Autodesk Inventor part; units mm, degrees
ref_plane "YZ Plane" through (0, 0, 0) normal (1, 0, 0) x (0, 1, 0)
ref_plane "XZ Plane" through (0, 0, 0) normal (0, 1, 0) x (-1, 0, 0)
ref_plane "XY Plane" through (0, 0, 0) normal (0, 0, 1) x (1, 0, 0)
sketch "Sketch1" plane through (0, 0, 0) normal (0, 0, 1) x (1, 0, 0)
  circle A0 centre (0, 0) radius 101.6
  circle A1 centre (0, 0) radius 14.2875
  dimension "d0" = 203.2
  dimension "d1" = 28.575
extrude "Extrusion1" add sketch "Sketch1" along normal blind 4.7625
sketch "Sketch4" plane through (0, 0, 4.7625) normal (0, 0, 1) x (1, 0, 0)
  circle A0 centre (0, 0) radius 101.6
  circle A1 centre (0, 92.075) radius 2.8063
  line L0 (0, 0) -> (0, 101.6) construction
  circle A2 centre (0, 0) radius 92.075 construction
  dimension "d58" = 9.525
extrude "Extrusion5" cut sketch "Sketch4" against normal through all contours A1
pattern_circular "Circular Pattern3" count 24 over 360 about axis through (0, 0, -10) along (0, 0, 1) of "Extrusion5"
sketch "Sketch6" plane through (0, 0, 4.7625) normal (0, 0, 1) x (1, 0, 0)
  circle A0 centre (0, 0) radius 101.6
  circle A1 centre (0, 23.8125) radius 2.3813
  circle A2 centre (0, 0) radius 23.8125 construction
  line L0 (0, 23.8125) -> (0, 0) construction
  dimension "d68" = 47.625
  dimension "d69" = 4.7625
extrude "Extrusion6" cut sketch "Sketch6" against normal through all contours A1
pattern_circular "Circular Pattern4" count 6 over 360 about axis through (0, 0, -10) along (0, 0, 1) of "Extrusion6"
sketch "Sketch7" plane through (0, 0, 4.7625) normal (0, 0, 1) x (1, 0, 0)
  circle A0 centre (-20.6222, -11.9062) radius 2.3813
  circle A1 centre (-20.6222, 11.9062) radius 2.3813
  circle A2 centre (0, 23.8125) radius 2.3813
  circle A3 centre (0, 0) radius 101.6
  line L0 (0, 0) -> (0, 23.8125) construction
  line L1 (0, 23.8125) -> (0, 0) construction
  line L2 (-20.6222, 11.9062) -> (0, 0) construction
  line L3 (-20.6222, -11.9062) -> (0, 0) construction
  line L4 (-25.4, 5.4993) -> (-68.7895, 30.5502)
  line L5 (-68.7895, -30.5502) -> (-25.4, -5.4993)
  arc A4 (-77.9615, 27.1385) -> (-77.9615, -27.1385) centre (0, 0) ccw
  arc A5 (-68.7895, 30.5502) -> (-77.9615, 27.1385) centre (-71.9645, 25.0509) ccw
  arc A6 (-77.9615, -27.1385) -> (-68.7895, -30.5502) centre (-71.9645, -25.0509) ccw
  arc A7 (-25.4, -5.4993) -> (-25.4, 5.4993) centre (-28.575, 0) ccw
  point P0 (-75.1279, -34.2097)
  point P1 (-75.1279, 34.2097)
  dimension "d75" = 19.05
  dimension "d76" = 6.35
  dimension "d78" = 7.9375
extrude "Extrusion7" cut sketch "Sketch7" against normal through all contours A7 L5 A6 A4 A5 L4
pattern_circular "Circular Pattern5" count 6 over 360 about axis through (0, 0, -10) along (0, 0, 1) of "Extrusion7"
properties part number "FlyWheelBase" material "Aluminum-6061"
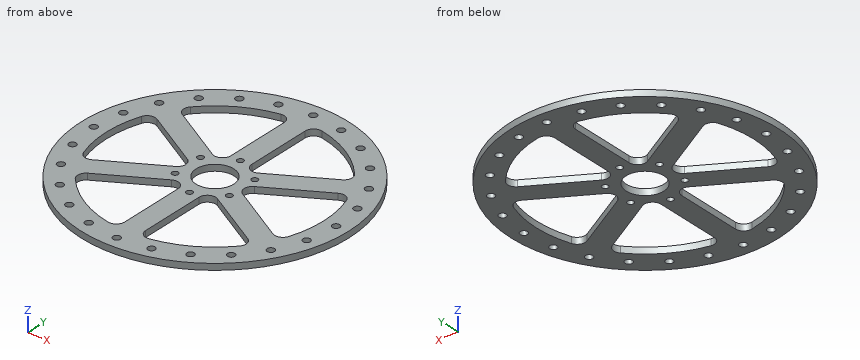
Geometry check sheet. Reference: the model listing, model coordinates, mm. Give positions to 0.01 mm unless a question says otherwise; leave off trailing zeros. Order: outer loops, then holes, each group sorted by start corner. A loop starts at its lowest first (then second) coordinate and runs counter-clockwise, first axis right, second up. Notation, with made-up numbers: M 8,47 L 60,47 A21 cw 60,55 Z; hole C -34.75,20 d9. An arc over 180 degrees is marked long. Use a Markdown table: item, result.
Item 1: Section check D-D (x = -36.5). Record the cut outline in (y, z).
Answers follow:
| item | result |
|---|---|
| outline | M -94.82,0 L -74.04,0 L -74.04,4.76 L -94.82,4.76 Z; M -30.24,0 L -11.91,0 L -11.91,4.76 L -30.24,4.76 Z; M 11.91,0 L 30.24,0 L 30.24,4.76 L 11.91,4.76 Z; M 74.04,0 L 94.82,0 L 94.82,4.76 L 74.04,4.76 Z |
Item 2: Material ranges on line 1 along Y through (x, z) = (-59.5, 2.3); line 2 along X through (y, z) = (-54, 2); line 3 along Y through (x, z) = (0, 2.25), recorded low to high.
Answers follow:
| item | result |
|---|---|
| line 1 | y = -82.35 to -57.22, -43.52 to -25.19, 25.19 to 43.52, 57.22 to 82.35 |
| line 2 | x = -86.06 to -62.44, -7.94 to 7.94, 62.44 to 86.06 |
| line 3 | y = -101.6 to -94.88, -89.27 to -26.19, -21.43 to -14.29, 14.29 to 21.43, 26.19 to 89.27, 94.88 to 101.6 |
Item 3: Section check A-A (x = 0). Record the cut outline in (y, z).
Answers follow:
| item | result |
|---|---|
| outline | M -101.6,0 L -94.88,0 L -94.88,4.76 L -101.6,4.76 Z; M -89.27,0 L -26.19,0 L -26.19,4.76 L -89.27,4.76 Z; M -21.43,0 L -14.29,0 L -14.29,4.76 L -21.43,4.76 Z; M 14.29,0 L 21.43,0 L 21.43,4.76 L 14.29,4.76 Z; M 26.19,0 L 89.27,0 L 89.27,4.76 L 26.19,4.76 Z; M 94.88,0 L 101.6,0 L 101.6,4.76 L 94.88,4.76 Z |
Item 4: Section check C-C (x = 30). Record the cut outline in (y, z), and give its area (3 significant figures).
Answers follow:
| item | result |
|---|---|
| outline | M -97.07,0 L -76.91,0 L -76.91,4.76 L -97.07,4.76 Z; M -26.49,0 L -8.16,0 L -8.16,4.76 L -26.49,4.76 Z; M 8.16,0 L 26.49,0 L 26.49,4.76 L 8.16,4.76 Z; M 76.91,0 L 97.07,0 L 97.07,4.76 L 76.91,4.76 Z |
| area | 367 mm2 |
Item 5: Depth check by flat-ended pin: P1, Ø1, axis at y = -7.5, z = 1.5, coming from the +X side; P2, Ø1.5, axis at y = -33, z = 4, coming from the -X side; P3, Ø2.5, axis at y = 62.5, z = 2.5, coming from the -X side. Enter the tip coordinate at first touch or a pass-through.
Answers follow:
| item | result |
|---|---|
| P1 | stops at x = 101.36 |
| P2 | stops at x = -96.35 |
| P3 | stops at x = -81.06 |
Item 6: Section check B-B (y = 0). Record the cut outline in (x, z).
Answers follow:
| item | result |
|---|---|
| outline | M -101.6,0 L -94.88,0 L -94.88,4.76 L -101.6,4.76 Z; M -89.27,0 L -82.55,0 L -82.55,4.76 L -89.27,4.76 Z; M -22.22,0 L -14.29,0 L -14.29,4.76 L -22.22,4.76 Z; M 14.29,0 L 22.22,0 L 22.22,4.76 L 14.29,4.76 Z; M 82.55,0 L 89.27,0 L 89.27,4.76 L 82.55,4.76 Z; M 94.88,0 L 101.6,0 L 101.6,4.76 L 94.88,4.76 Z |
